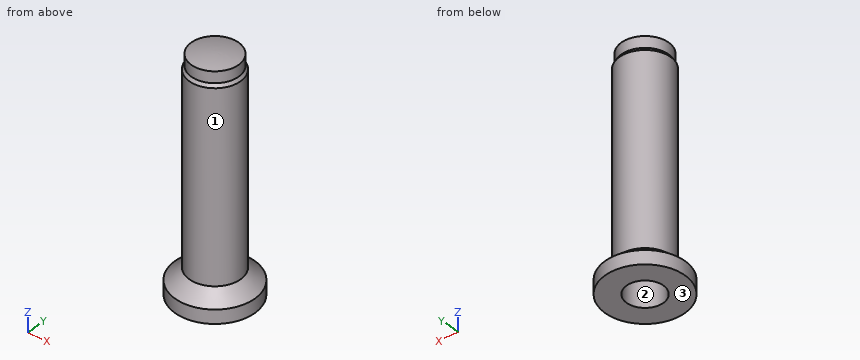
from build123d import *


with BuildPart() as f1:
    # F0 (on Front) → F1 (revolve)
    with BuildSketch(Plane.XZ):
        with BuildLine():
            ThreePointArc((13.845299, 133.575579), (6.95919, 134.642957), (0, 135))
            Line((0, 135), (0, 125))
            Line((0, 125), (10.75, 125))
            Line((10.75, 125), (10.75, 0))
            Line((10.75, 0), (23.342275, 0))
            Line((23.342275, 0), (23.342275, 8))
            Line((23.342275, 8), (15, 15))
            Line((15, 15), (15, 125))
            Line((15, 125), (13.845299, 127))
            Line((13.845299, 127), (13.845299, 133.575579))
        make_face()
    revolve(axis=Axis((0, 0, 8.877954), (0, 0, -1)))


solid = f1.part
Can you work these out from the model? Positions are in its coordinate system, mm. Face numbers are marked on the shaded views. Round coordinates to 2 decimals unless told otherwise and drop trailing zeros. Loops run counter-clockwise (first coordinate to the right, second up) from the corner with the lowest first, then second, coordinate; pieces in that order, holes last. Notation, with made-up numbers: (-26.5, -27.5) - (-8.5, -27.5) arc R29 ccw to (-8.5, -7.5) - close; hole circle Ø7 at (-28.75, 66). An arc over 180 degrees is marked (long way). Answer in a Markdown table with one row per item. Add a question column.
Q1. I want a section at A-A on z = 36.5. List the corners of the cut face in (x, y) for me.
Q2. For pin 1 Ø6 at (x, y) = (-2, -14.5) entering from -Z; pin 2 Ø10 at (y, z) = (-17.5, 99.5) entering from -X; pin 3 Ø2 at (y, z) = (4.5, 32.5) entering from -X; pin 4 Ø8 at (x, y) = (-1, 0) entering from -Z, each with a flat end and sliding along its axis, tell me the tip position at first contact or that it passes through.
Q3. We'd pull the mould along X, two halves only. Please class the marked faces 1, 2 and 3: pulls with the +X half, pulls with the -X half, needs draft (parallel to the pull), parting line crosses it, or undercut.
Q4. I need wall thicknesses on L1, parallel to X at y = 0, z = 95; L2, parallel to Y at x = -6, z = 29. Which ranges of each line are inside material? Lowest first, please.
A:
| question | item | result |
|---|---|---|
| 1 | outline | circle Ø30 at (0, 0); hole circle Ø21.5 at (0, 0) |
| 2 | pin 1 | z = 0 |
| 2 | pin 2 | x = -8.29 |
| 2 | pin 3 | x = -14.59 |
| 2 | pin 4 | z = 125 |
| 3 | face 1 | parting line crosses it |
| 3 | face 2 | undercut |
| 3 | face 3 | needs draft |
| 4 | L1 | -15 to -10.75, 10.75 to 15 |
| 4 | L2 | -13.75 to -8.92, 8.92 to 13.75 |
